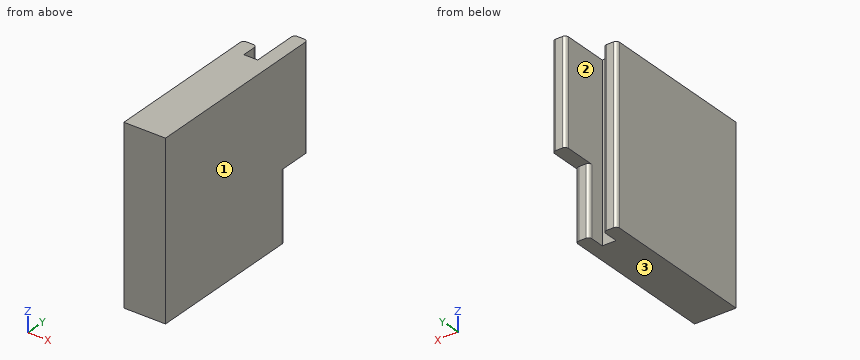
from build123d import *

# Parameters (mm, degrees)
BOSS_EXTRU_1_DEPTH = 25
CONG_1_R           = 0.5
ESQUISSE2_W        = 15
ESQUISSE2_H        = 5
BOSS_EXTRU_2_DEPTH = 2
CONG_2_R           = 0.5


with BuildPart() as part:
    # Esquisse1 → Boss.-Extru.1 (new body)
    with BuildSketch(Plane.XY):
        Polygon((-4.120689655, 2.5), (-2.120689655, 2.5), (-2.120689655, 0), (-0.120689655, 0), (-0.120689655, 2.5), (1.879310345, 2.5), (1.879310345, -20.5), (-4.120689655, -20.5), align=None)
    extrude(amount=BOSS_EXTRU_1_DEPTH)

    # Congé1
    cong_1_edges = [part.edges().sort_by_distance(p)[0] for p in [
        (-4.120689655, 2.5, 12.5),
        (-2.120689655, 2.5, 12.5),
        (-0.120689655, 2.5, 12.5),
        (1.879310345, 2.5, 12.5),
    ]]
    fillet(cong_1_edges, radius=CONG_1_R)

    # Esquisse2 → Boss.-Extru.2 (add)
    with BuildSketch(Plane(origin=(1.879310345, 0, 0), x_dir=(0, 0, -1), z_dir=(1, 0, 0))):
        with Locations((-17.5, 4.5)):
            Rectangle(ESQUISSE2_W, ESQUISSE2_H)
    extrude(amount=-BOSS_EXTRU_2_DEPTH)

    # Congé2
    cong_2_edges = [part.edges().sort_by_distance(p)[0] for p in [
        (-0.120689655, 7, 17.5),
        (1.879310345, 7, 17.5),
    ]]
    fillet(cong_2_edges, radius=CONG_2_R)


solid = part.part
The listing builds one solid part. Answer for the finished solid, in the listing's coordinates (mm). Face numbers are marked on the shaded views. Give positions to 0.01 mm unless a question says otherwise; leave off trailing zeros. Loops run counter-clockwise (first coordinate to the right, second up) from the corner with the lowest first, then second, coordinate; pieces in that order, holes last. Notation, with made-up numbers: M 65,-15 L 69,-15 A16 cw 69,15 Z; hole C 56.5,1 d5. An arc over 180 degrees is marked long. Answer as CSV lines item,"result".
Item 1: The part is cut by section D-D (y = 4.5). Give the vertices of the cut face in (x, z).
Values follow:
outline,"M -0.12,10 L 1.88,10 L 1.88,25 L -0.12,25 Z"
Item 2: The part is cut by section A-A (y = 1.25). Give the vertices of the cut face in (x, z), and give its area (3 significant figures).
Values follow:
outline,"M -4.12,0 L -2.12,0 L -2.12,25 L -4.12,25 Z; M -0.12,0 L 1.88,0 L 1.88,25 L -0.12,25 Z"
area,"100 mm^2"
Item 3: Given pin 1 Ø0.6 at (x, y) = (0.5, 4.5) entering from -Z, flat-ended and moving along its own axis, determine where the tip first touches the part or whether it passes through.
Values follow:
pin 1,"stops at z = 10"
Item 4: The part is cut by section C-C (x = -0.65). Give the vertices of the cut face in (y, z), and give its area (4 significant figures).
Values follow:
outline,"M -20.5,0 L 0,0 L 0,25 L -20.5,25 Z"
area,"512.5 mm^2"
Item 5: The mould has two halves that part along X. Classify the marked faces 1, 2 and 3: released by +X, released by -X, zero draft, split by the parting line, or undercut.
Values follow:
face 1,"released by +X"
face 2,"undercut"
face 3,"zero draft"
Item 6: Straight lines are drawn through the part: line 1 along X through (y, z) = (0.75, 21); line 2 along Y through (x, z) = (-2, 13.5); line 3 along Z through (x, y) = (1.5, 6). For each, find the intervals that lie inside material, in ascending order. Write a range as [from, to].
Values follow:
line 1,"x = [-4.12, -2.12], [-0.12, 1.88]"
line 2,"y = [-20.5, 0]"
line 3,"z = [10, 25]"
Item 7: The part is cut by section B-B (z = 1.5). Give the vertices of the cut face in (x, y).
Values follow:
outline,"M -4.12,-20.5 L 1.88,-20.5 L 1.88,2 A0.5 ccw 1.38,2.5 L 0.38,2.5 A0.5 ccw -0.12,2 L -0.12,0 L -2.12,0 L -2.12,2 A0.5 ccw -2.62,2.5 L -3.62,2.5 A0.5 ccw -4.12,2 Z"
